Geometry check sheet. Reference: the model listing, model coordinates, mm. A direction names the side the tool comes from. Round coordinates to 2 decimals unless told otherwise and drop trailing zeros. Write each loop counter-clockwise with the first axis right and the second up, starting at its lowest first coordinate (ties: lowest second). Pieces come first, ordered by that corner, then holes.
Item 1: Access from +Z, -Z, +X, -X, +Y, -Y to the whole of each face (thin tool, end or side, straight path). Record for faces 5 (the face through (-10, 5, 32.75)), 6 (the face through (-2.38, -10.74, 35.54)), 7 (the face through (-3.4, 12.3, 32.5)).
Item 2: Cross-section at C-C (z = 20). Enter the section's corners in (x, y).
Item 3: Cross-section at D-D (z = 14.5). Enter the section's corners in (x, y).
Item 4: Cross-section at B-B (x = 0). State how many separate pieces and enclosed holes the cut face has, then the cut area to 3 significant figures.
Item 5: Scan lines: probe 1 along Z at (x, y) = (0, -11.6); probe 2 along Y at (x, z) = (0, 36.1); probe 3 along Z at (x, y) = (8.5, -11.25). Record each from-to range of solid material in increasing order.
Item 6: Depth check by flat-ended pin: P1, Ø1.5, axis at y = -5, z = 26, coming from the -X side; P2, Ø1.6, axis at x = 0, z = 20, coming from the -Y side; P3, Ø3, axis at y = -7, z = 30.5, coming from the +X side; P4, Ø9, axis at x = -5.5, y = 0.5, coming from the +Z side. Enter the tip coordinate at first touch or a pass-through.
Item 7: Cross-section at A-A (z = 7.5). Enter the section's corners in (x, y), then the cut area to 3 significant figures.
Item 8: Draft check along X on faces 1 (the face through (-10.316, -7.91, 35.342)), 2 (the face through (1, -11, 20)), 3 (the face through (8, -3, 32.75)), 4 (the face through (6.2, -6.2, 0)). Enter one of: pulls with the +X half, pulls with the -X half, needs draft (parallel to the pull), parting line crosses it, or undercut.
from build123d import *

# Parameters (mm, degrees)
SKETCH1_R           = 14.5
BOSS_EXTRUDE1_DEPTH = 4
SKETCH2_R           = 15
BOSS_EXTRUDE2_DEPTH = 8
SKETCH3_R           = 13
BOSS_EXTRUDE3_DEPTH = 16
SKETCH4_R           = 15
BOSS_EXTRUDE4_DEPTH = 4.5
SKETCH5_R           = 12.5
BOSS_EXTRUDE5_DEPTH = 0.5
SKETCH6_R           = 13
BOSS_EXTRUDE6_DEPTH = 5.25
SKETCH7_R           = 11
CUT_EXTRUDE1_DEPTH  = 5.5
SKETCH8_R           = 10
CUT_EXTRUDE2_DEPTH  = 32.75
FILLET1_R           = 0.75
CHAMFER1_SIZE       = 0.5
SKETCH11_W          = 1
SKETCH11_H          = 15


with BuildPart() as part:
    # Sketch1 → Boss-Extrude1 (new body)
    with BuildSketch(Plane.XY):
        Circle(SKETCH1_R)
    extrude(amount=BOSS_EXTRUDE1_DEPTH)

    # Sketch2 → Boss-Extrude2 (add)
    with BuildSketch(Plane.XY.offset(4)):
        Circle(SKETCH2_R)
    extrude(amount=BOSS_EXTRUDE2_DEPTH)

    # Sketch3 → Boss-Extrude3 (add)
    with BuildSketch(Plane.XY.offset(12)):
        Circle(SKETCH3_R)
    extrude(amount=BOSS_EXTRUDE3_DEPTH)

    # Sketch4 → Boss-Extrude4 (add)
    with BuildSketch(Plane.XY.offset(28)):
        Circle(SKETCH4_R)
    extrude(amount=BOSS_EXTRUDE4_DEPTH)

    # Sketch5 → Boss-Extrude5 (add)
    with BuildSketch(Plane.XY.offset(32.5)):
        Circle(SKETCH5_R)
    extrude(amount=BOSS_EXTRUDE5_DEPTH)

    # Sketch6 → Boss-Extrude6 (add)
    with BuildSketch(Plane.XY.offset(33)):
        Circle(SKETCH6_R)
    extrude(amount=BOSS_EXTRUDE6_DEPTH)

    # Sketch7 → Cut-Extrude1 (cut)
    with BuildSketch(Plane.XY.offset(38.25)):
        Circle(SKETCH7_R)
    extrude(amount=-CUT_EXTRUDE1_DEPTH, mode=Mode.SUBTRACT)

    # Sketch8 → Cut-Extrude2 (cut)
    with BuildSketch(Plane.XY.offset(32.75)):
        with Locations((-1.44, 0.75)):
            Circle(SKETCH8_R)
    extrude(amount=-CUT_EXTRUDE2_DEPTH, mode=Mode.SUBTRACT)

    # Fillet1
    fillet1_edges = [part.edges().sort_by_distance(p)[0] for p in [
        (-13, 0, 12),
        (-13, 0, 28),
    ]]
    fillet(fillet1_edges, radius=FILLET1_R)

    # Chamfer1
    chamfer1_edges = [part.edges().sort_by_distance(p)[0] for p in [
        (-13, 0, 38.25),
    ]]
    chamfer(chamfer1_edges, length=CHAMFER1_SIZE)

    # Sketch11 → Ø2.0 (2) Diameter Hole2 (revolve, cut)
    with BuildSketch(Plane(origin=(0, 0, 20), x_dir=(0, 0, 1), z_dir=(1, 0, 0))):
        with Locations((0.5, 7.5)):
            Rectangle(SKETCH11_W, SKETCH11_H)
    revolve(axis=Axis((0, 6.35, 20), (0, -1, 0)), mode=Mode.SUBTRACT)


solid = part.part
Resolved:
1. face 5: -Z
1. face 6: +Z
1. face 7: none
2. outline: (-1, -12.96) - (-1, -9.24) arc R10 cw (long way) to (1, -8.95) - (1, -12.96) arc R13 ccw (long way) to start
3. outline: circle Ø26 at (0, 0); hole circle Ø20 at (-1.44, 0.75)
4. separate pieces: 3
4. enclosed holes: 0
4. area: 279 mm2
5. probe 1: z = 0 to 19, 21 to 38.25
5. probe 2: y = -13 to -11, 11 to 13
5. probe 3: z = 0 to 12, 28 to 32.5
6. P1: stops at x = -12.29
6. P2: stops at y = 10.5
6. P3: stops at x = 13.96
6. P4: passes through
7. outline: circle Ø30 at (0, 0); hole circle Ø20 at (-1.44, 0.75)
7. area: 393 mm2
8. face 1: parting line crosses it
8. face 2: undercut
8. face 3: undercut
8. face 4: needs draft
